Here's how the part is built. I have some questions about the finished solid (model axes, mm). A direction names the side the tool comes from. Round coordinates to 2 decimals unless told otherwise and drop trailing zeros. Loops run counter-clockwise (first coordinate to the right, second up) from the corner with the lowest first, then second, coordinate; pieces in that order, holes last. Notation, with made-up numbers: M -8,53.5 L 17,53.5 A20 ccw 17,83.5 Z; hole C 53,40 d11. An arc over 180 degrees is marked long. Answer as a JSON object with one key per item and string values.
from build123d import *

# Parameters (mm, degrees)
SZKIC1_R                      = 12
DODANIE_WYCI_GNI_CIE2_DEPTH   = 4
SZKIC1_R_2                    = 4.5
DODANIE_WYCI_GNI_CIE2_2_DEPTH = 4
DODANIE_WYCI_GNI_CIE3_DEPTH   = 4
WYTNIJ_WYCI_GNI_CIE1_REACH    = 40.63
SZKIC3_R                      = 1.5
SZKIC4_R                      = 4.1
SZKIC4_R_2                    = 2.6
DODANIE_WYCI_GNI_CIE4_DEPTH   = 15
SZKIC5_W                      = 20
SZKIC5_H                      = 2
DODANIE_WYCI_GNI_CIE5_DEPTH   = 15
SZKIC6_W                      = 16
SZKIC6_H                      = 0.4
WYTNIJ_WYCI_GNI_CIE2_DEPTH    = 15
SZKIC7_W                      = 6.95515277
SZKIC7_H                      = 2.2
SZKIC7_W_2                    = 6.645937882
DODANIE_WYCI_GNI_CIE6_DEPTH   = 15
SZKIC10_R                     = 1.5
WYTNIJ_WYCI_GNI_CIE4_DEPTH    = 5


with BuildPart() as part:
    # Szkic1 → Dodanie-wyci_gni_cie2 (new body)
    with BuildSketch(Plane.XY):
        Circle(SZKIC1_R)
    extrude(amount=DODANIE_WYCI_GNI_CIE2_DEPTH)



with BuildPart() as body_2:
    # Szkic1 → Dodanie-wyci_gni_cie2 2 (new body)
    with BuildSketch(Plane.XY):
        with Locations((0, 32)):
            Circle(SZKIC1_R_2)
    extrude(amount=DODANIE_WYCI_GNI_CIE2_2_DEPTH)


with BuildPart() as part_1:
    add(part.part)

    add(body_2.part)  # Dodanie-wyci_gni_cie3 merges body 2
    # Szkic2 → Dodanie-wyci_gni_cie3 (add)
    with BuildSketch(Plane(origin=(0, 0, 0), x_dir=(-1, 0, 0), z_dir=(0, 0, -1))):
        Polygon((-4.5, 32), (-12, 0), (12, 0), (4.5, 32), align=None)
    extrude(amount=-DODANIE_WYCI_GNI_CIE3_DEPTH)

    # Szkic3 → Wytnij-wyci_gni_cie1 (cut, up to next)
    with BuildSketch(Plane(origin=(0, 0, 0), x_dir=(-1, 0, 0), z_dir=(0, 0, -1)), mode=Mode.PRIVATE) as wytnij_wyci_gni_cie1_sk1:
        with Locations((0, 32)):
            Circle(SZKIC3_R)
    wytnij_wyci_gni_cie1_tool1 = extrude(wytnij_wyci_gni_cie1_sk1.sketch, amount=-WYTNIJ_WYCI_GNI_CIE1_REACH, mode=Mode.PRIVATE) & part_1.part
    # Szkic3 → Wytnij-wyci_gni_cie1 (cut, up to next)
    with BuildSketch(Plane(origin=(0, 0, 0), x_dir=(-1, 0, 0), z_dir=(0, 0, -1)), mode=Mode.PRIVATE) as wytnij_wyci_gni_cie1_sk2:
        with Locations((0, 28)):
            Circle(SZKIC3_R)
    wytnij_wyci_gni_cie1_tool2 = extrude(wytnij_wyci_gni_cie1_sk2.sketch, amount=-WYTNIJ_WYCI_GNI_CIE1_REACH, mode=Mode.PRIVATE) & part_1.part
    # Szkic3 → Wytnij-wyci_gni_cie1 (cut, up to next)
    with BuildSketch(Plane(origin=(0, 0, 0), x_dir=(-1, 0, 0), z_dir=(0, 0, -1)), mode=Mode.PRIVATE) as wytnij_wyci_gni_cie1_sk3:
        with Locations((0, 24)):
            Circle(SZKIC3_R)
    wytnij_wyci_gni_cie1_tool3 = extrude(wytnij_wyci_gni_cie1_sk3.sketch, amount=-WYTNIJ_WYCI_GNI_CIE1_REACH, mode=Mode.PRIVATE) & part_1.part
    # Szkic3 → Wytnij-wyci_gni_cie1 (cut, up to next)
    with BuildSketch(Plane(origin=(0, 0, 0), x_dir=(-1, 0, 0), z_dir=(0, 0, -1)), mode=Mode.PRIVATE) as wytnij_wyci_gni_cie1_sk4:
        with Locations((0, 20)):
            Circle(SZKIC3_R)
    wytnij_wyci_gni_cie1_tool4 = extrude(wytnij_wyci_gni_cie1_sk4.sketch, amount=-WYTNIJ_WYCI_GNI_CIE1_REACH, mode=Mode.PRIVATE) & part_1.part
    add(wytnij_wyci_gni_cie1_tool1.solids().sort_by_distance((0, 32, 0))[0], mode=Mode.SUBTRACT)
    add(wytnij_wyci_gni_cie1_tool2.solids().sort_by_distance((0, 28, 0))[0], mode=Mode.SUBTRACT)
    add(wytnij_wyci_gni_cie1_tool3.solids().sort_by_distance((0, 24, 0))[0], mode=Mode.SUBTRACT)
    add(wytnij_wyci_gni_cie1_tool4.solids().sort_by_distance((0, 20, 0))[0], mode=Mode.SUBTRACT)

    # Szkic4 → Dodanie-wyci_gni_cie4 (add)
    with BuildSketch(Plane.XY.offset(4)):
        Circle(SZKIC4_R)
        Circle(SZKIC4_R_2, mode=Mode.SUBTRACT)
    extrude(amount=DODANIE_WYCI_GNI_CIE4_DEPTH)

    # Szkic5 → Dodanie-wyci_gni_cie5 (add)
    with BuildSketch(Plane.XY.offset(4)):
        with Locations((0, -3)):
            Rectangle(SZKIC5_W, SZKIC5_H)
    extrude(amount=DODANIE_WYCI_GNI_CIE5_DEPTH)

    # Szkic6 → Wytnij-wyci_gni_cie2 (cut)
    with BuildSketch(Plane.XY.offset(4)):
        with Locations((-2, -1.8)):
            Rectangle(SZKIC6_W, SZKIC6_H)
    extrude(amount=WYTNIJ_WYCI_GNI_CIE2_DEPTH, mode=Mode.SUBTRACT)

    # Szkic7 → Dodanie-wyci_gni_cie6 (add)
    with BuildSketch(Plane.XY.offset(4)):
        with Locations((-6.522423615, -0.5)):
            Rectangle(SZKIC7_W, SZKIC7_H)
        with Locations((6.677031059, -0.5)):
            Rectangle(SZKIC7_W_2, SZKIC7_H)
    extrude(amount=DODANIE_WYCI_GNI_CIE6_DEPTH)

    # Szkic10 → Wytnij-wyci_gni_cie4 (cut)
    with BuildSketch(Plane(origin=(0, 0.6, 0), x_dir=(1, 0, 0), z_dir=(0, 1, 0))):
        with Locations(Location((-7, -12, 0), (0, 0, 180))):
            Circle(SZKIC10_R)
        with Locations(Location((7, -12, 0), (0, 0, 180))):
            Circle(SZKIC10_R)
    extrude(amount=-WYTNIJ_WYCI_GNI_CIE4_DEPTH, mode=Mode.SUBTRACT)


solid = part_1.part
Item 1: I want a section at D-D, the plane x = -7.25. Please give me the cut outline in (y, z).
Resolved:
{"outline": "M -9.56,0 L 20.27,0 L 20.27,4 L 0.6,4 L 0.6,10.52 L -1.6,10.52 L -1.6,4 L -2,4 L -2,10.52 L -4,10.52 L -4,4 L -9.56,4 Z; M -4,13.48 L -2,13.48 L -2,19 L -4,19 Z; M -1.6,13.48 L 0.6,13.48 L 0.6,19 L -1.6,19 Z"}
Item 2: I'm going to push flat-ended pins straight in: pin 1 Ø2.5 at (x, y) = (0, 32) entering from -Z; pin 2 Ø5 at (x, z) = (-7, 12) entering from -Y; pin 3 Ø0.6 at (y, z) = (-3, 14.5) entering from +X; pin 4 Ø1.1 at (y, z) = (-0.5, 8.5) entering from -X. Where does each tip first touch, or does it pass through?
Resolved:
{"pin 1": "through", "pin 2": "y = -4", "pin 3": "x = 10", "pin 4": "x = -10"}
Item 3: I want a section at A-A, the plane z = 12. State how many separate pieces and enclosed holes the cut face has, then the cut area to 3 significant figures.
Resolved:
{"separate pieces": "6", "enclosed holes": "0", "area": "62.0 mm²"}
Item 4: I want a section at B-B, the plane z = 5.25. Please give me the cut outline in (x, y), then the cut area to 3 significant figures.
Resolved:
{"outline": "M -10,-4 L -0.9,-4 A4.1 ccw 0.9,-4 L 10,-4 L 10,-2 L -10,-2 Z; M -10,-1.6 L -2.05,-1.6 A2.6 cw long 2.05,-1.6 L 10,-1.6 L 10,0.6 L 4.06,0.6 A4.1 ccw -4.06,0.6 L -10,0.6 Z", "area": "87.2 mm²"}
Item 5: Please list where these lines run through material, in increasing order: probe 1 along Y at (x, z) = (-6.75, 14.5); probe 2 along Z at (x, y) = (7, -3.2); probe 3 along Y at (x, z) = (0, 9.25). Write a range as from..to.
Resolved:
{"probe 1": "-4..-2, -1.6..0.6", "probe 2": "0..10.5, 13.5..19", "probe 3": "-4.1..-2, 2.6..4.1"}
Item 6: On a 3-axis mill with a long thin cutter (end or side, diameter ignored), from which of +Z, -Z, +X, -X, +Y, -Y can I reach the whole of each face in a straight line? I mean faces 1 (the face through (7, 0.6, 10)), 2 (the face through (-5, -4, 11)), 3 (the face through (5, -4, 11)). Say none if no direction works.
Resolved:
{"face 1": "+Z, +X, +Y", "face 2": "+Z, -X, -Y", "face 3": "+Z, +X, -Y"}
Item 7: If we mould it in two halves opening along X, with no side actions, what happens to faces 4 (the face through (-5, -1.6, 11)), 5 (the face through (-10, -3, 11)), 6 (the face through (8.5, -0.48, 12.07)), 7 (the face through (10, -1, 11))? For each: pulls with the +X half, pulls with the -X half, needs draft (parallel to the pull), parting line crosses it, or undercut.
Resolved:
{"face 4": "needs draft", "face 5": "pulls with the -X half", "face 6": "undercut", "face 7": "pulls with the +X half"}
Item 8: I want a section at C-C, the plane y = 28. Please give me the cut outline in (x, z).
Resolved:
{"outline": "M -5.44,0 L -1.5,0 L -1.5,4 L -5.44,4 Z; M 1.5,0 L 5.44,0 L 5.44,4 L 1.5,4 Z"}
